Autodesk Inventor part; units mm, degrees
ref_plane "YZ Plane" through (0, 0, 0) normal (1, 0, 0) x (0, 1, 0)
ref_plane "XZ Plane" through (0, 0, 0) normal (0, 1, 0) x (-1, 0, 0)
ref_plane "XY Plane" through (0, 0, 0) normal (0, 0, 1) x (1, 0, 0)
sketch "Sketch1" plane through (0, 0, 0) normal (0, 1, 0) x (-1, 0, 0)
  line L0 (76, -4.8141) -> (76, 4.8141)
  line L1 (-76, 4.8141) -> (-76, -4.8141)
  circle A0 centre (0, 0) radius 14
  line L2 (-23, 5) -> (-20, 5)
  line L3 (-20, 5) -> (-20, -5)
  line L4 (-20, -5) -> (-23, -5)
  line L5 (-23, -5) -> (-23, 5)
  line L6 (20, 5) -> (23, 5)
  line L7 (23, 5) -> (23, -5)
  line L8 (23, -5) -> (20, -5)
  line L9 (20, -5) -> (20, 5)
  line L10 (-73, 5) -> (-70, 5)
  line L11 (-70, 5) -> (-70, -5)
  line L12 (-70, -5) -> (-73, -5)
  line L13 (-73, -5) -> (-73, 5)
  line L14 (70, 5) -> (73, 5)
  line L15 (73, 5) -> (73, -5)
  line L16 (73, -5) -> (70, -5)
  line L17 (70, -5) -> (70, 5)
  arc A1 (-13, -18) -> (-19, -18) centre (-16, -18) ccw
  arc A2 (-19, 18) -> (-13, 18) centre (-16, 18) ccw
  arc A3 (19, -18) -> (13, -18) centre (16, -18) ccw
  arc A4 (13, 18) -> (19, 18) centre (16, 18) ccw
  line L18 (-19, 18) -> (-19, 21)
  line L19 (-13, 18) -> (-13, 21)
  line L20 (13, 18) -> (13, 21)
  line L21 (19, 18) -> (19, 21)
  line L22 (13, -18) -> (13, -21)
  line L23 (19, -18) -> (19, -21)
  line L24 (-13, -18) -> (-13, -21)
  line L25 (-19, -18) -> (-19, -21)
  line L26 (-13, -21) -> (13, -21)
  line L27 (13, 21) -> (-13, 21)
  arc A5 (-53, 18) -> (-47, 18) centre (-50, 18) ccw
  arc A6 (-47, -18) -> (-53, -18) centre (-50, -18) ccw
  arc A7 (47, 18) -> (53, 18) centre (50, 18) ccw
  arc A8 (53, -18) -> (47, -18) centre (50, -18) ccw
  line L28 (-53, 18) -> (-53, 21)
  line L29 (-47, 18) -> (-47, 21)
  line L30 (-53, -18) -> (-53, -21)
  line L31 (-47, -18) -> (-47, -21)
  line L32 (53, -18) -> (53, -21)
  line L33 (47, -18) -> (47, -21)
  line L34 (53, 18) -> (53, 21)
  line L35 (47, 18) -> (47, 21)
  line L36 (71.3401, 21) -> (53, 21)
  line L37 (47, 21) -> (19, 21)
  line L38 (19, -21) -> (47, -21)
  line L39 (53, -21) -> (71.3401, -21)
  line L40 (-71.3401, -21) -> (-53, -21)
  line L41 (-47, -21) -> (-19, -21)
  line L42 (-19, 21) -> (-47, 21)
  line L43 (-53, 21) -> (-71.3401, 21)
  line L44 (-75.9657, 5.1827) -> (-73.3059, 19.3686)
  line L45 (-73.3059, -19.3686) -> (-75.9657, -5.1827)
  line L46 (73.3059, 19.3686) -> (75.9657, 5.1827)
  line L47 (73.3059, -19.3686) -> (75.9657, -5.1827)
  arc A9 (-71.3401, 21) -> (-73.3059, 19.3686) centre (-71.3401, 19) ccw
  arc A10 (-75.9657, 5.1827) -> (-76, 4.8141) centre (-74, 4.8141) ccw
  arc A11 (-76, -4.8141) -> (-75.9657, -5.1827) centre (-74, -4.8141) ccw
  arc A12 (-73.3059, -19.3686) -> (-71.3401, -21) centre (-71.3401, -19) ccw
  arc A13 (71.3401, -21) -> (73.3059, -19.3686) centre (71.3401, -19) ccw
  arc A14 (75.9657, -5.1827) -> (76, -4.8141) centre (74, -4.8141) ccw
  arc A15 (73.3059, 19.3686) -> (71.3401, 21) centre (71.3401, 19) ccw
  arc A16 (76, 4.8141) -> (75.9657, 5.1827) centre (74, 4.8141) ccw
  point P0 (-73, -21)
  point P1 (73, 21)
  point P2 (73, -21)
  point P3 (-73, 21)
  point P4 (-20, 0)
  point P5 (20, 0)
  point P6 (-76, 5)
  point P7 (-76, -5)
  point P8 (76, 5)
  point P9 (76, -5)
  dimension "d2" = 42
  dimension "d3" = 28
  dimension "d4" = 76
  dimension "d6" = 3
  dimension "d7" = 10
  dimension "d8" = 20
  dimension "d9" = 3
  dimension "d10" = 10
  dimension "d11" = 20
  dimension "d12" = 3
  dimension "d13" = 10
  dimension "d14" = 3
  dimension "d15" = 3
  dimension "d16" = 10
  dimension "d17" = 3
  dimension "d18" = 5
  dimension "d19" = 5
  dimension "d20" = 6
  dimension "d21" = 16
  dimension "d24" = 6
  dimension "d25" = 16
  dimension "d26" = 6
  dimension "d27" = 16
  dimension "d28" = 6
  dimension "d29" = 16
  dimension "d32" = 6
  dimension "d33" = 50
  dimension "d35" = 50
  dimension "d38" = 76
  dimension "d39" = 21
  dimension "d40" = 3
  dimension "d41" = 3
  dimension "d42" = 10
  dimension "d43" = 10
  dimension "d44" = 21
  dimension "d45" = 2
  dimension "d46" = 50
  dimension "d47" = 50
  dimension "d48" = 3
  dimension "d49" = 3
  dimension "d50" = 3
  dimension "d51" = 3
  dimension "d52" = 3
  dimension "d53" = 3
  dimension "d54" = 3
  dimension "d55" = 3
  dimension "d56" = 100.62
extrude "Extrusion1" add sketch "Sketch1" along normal blind 3
properties part number "Camera Platform"
Geometry check sheet. Reference: the model listing, model coordinates, mm. A direction names the side the tool comes from. Coordinates: 2 decimals unless noted, no trailing zeros. Loops run counter-clockwise (first coordinate to the right, second up) from the corner with the lowest first, then second, coordinate; pieces in that order, holes last.
Item 1: Release check for a two-part mould opening along X. For faces 5 (the face through (13, 1, 19)), 6 (the face through (0, 1, 21)), 7 (the face through (74.654, 1.479, 12.176)) record: released by +X, released by -X, zero draft, split by the parting line, or undercut.
Item 2: Thickness scan on line 1 (Z direction, x = 0, y = 1.45); line 2 (X direction, y = 2, z = -17.5); line 3 (X direction, y = 2.7, z = -1). Record the ranges inside material, lowest first.
Item 3: Sectioned sample at B-B, the plane z = 3.5. Record the boundary of the cut face in (x, y), then the cut area to 3 significant figures.
Item 4: Access from +Z, -Z, +X, -X, +Y, -Y to the whole of each face (thin tool, end or side, straight path). Record for faces 1 (the face through (1.1, 0, 14.3)), 2 (the face through (19, 1, -19)), 3 (the face through (73, 1, 0)), 4 (the face through (19, 1, 19)).
Item 5: Go/stop test with flat-tipped pins: pin 1 Ø0.9 at (y, z) = (1, -19) entering from +X; pin 2 Ø6 at (x, z) = (-41, 14.5) entering from -Y; pin 3 Ø0.9 at (y, z) = (1, -20) entering from -X; pin 4 Ø1.5 at (y, z) = (1.5, -19) entering from -X. Record where each tip stops, or that it passes through.
Item 6: Sectioned sample at A-A, the plane x = 0. Record the boundary of the cut face in (y, z).
Item 7: Sectioned sample at C-C, the plane y = 1.2. Count the separate pieces of the cut face and the enclosed holes in it, then the cut area to 3 significant figures.
Item 8: Sectioned sample at D-D, the plane x = -50. Record the boundary of the cut face in (y, z), then the cut area to 3 significant figures.
Check result:
1. face 5: undercut
1. face 6: zero draft
1. face 7: released by +X
2. line 1: z = -21 to -14, 14 to 21
2. line 2: x = -73.66 to -52.96, -47.04 to -18.96, -13.04 to 13.04, 18.96 to 47.04, 52.96 to 73.66
2. line 3: x = -76 to -73, -70 to -23, -20 to -13.96, 13.96 to 20, 23 to 70, 73 to 76
3. outline: (-76, 0) - (-73, 0) - (-73, 3) - (-76, 3) - close; (-70, 0) - (-23, 0) - (-23, 3) - (-70, 3) - close; (-20, 0) - (-13.56, 0) - (-13.56, 3) - (-20, 3) - close; (13.56, 0) - (20, 0) - (20, 3) - (13.56, 3) - close; (23, 0) - (70, 0) - (70, 3) - (23, 3) - close; (73, 0) - (76, 0) - (76, 3) - (73, 3) - close
3. area: 339 mm2
4. face 1: +Z, -Z, +X, -X, -Y
4. face 2: -Z, +Y, -Y
4. face 3: +Y, -Y
4. face 4: +Z, +Y, -Y
5. pin 1: stops at x = 73.46
5. pin 2: stops at y = 0
5. pin 3: stops at x = -73.26
5. pin 4: stops at x = -73.52
6. outline: (0, -21) - (3, -21) - (3, -14) - (0, -14) - close; (0, 14) - (3, 14) - (3, 21) - (0, 21) - close
7. separate pieces: 1
7. enclosed holes: 5
7. area: 5,290 mm2
8. outline: (0, -15) - (3, -15) - (3, 15) - (0, 15) - close
8. area: 90.0 mm2
